Source: CAD feature listing. Evaluate the final solid. Frame: model axes, mm. A direction names the side the tool comes from. Give positions to 0.01 mm unless a question says otherwise; leave off trailing zeros. Order: outer loops, then holes, each group sorted by start corner. A loop starts at its lowest first (then second) coordinate and runs counter-clockwise, first axis right, second up.
from build123d import *

# Parameters (mm, degrees)
F0_R     = 40
F1_DEPTH = 120
F2_R     = 2.65
F3_DEPTH = 10
F4_R     = 2.25
F5_DEPTH = 25
F6_R     = 37.5
F7_DEPTH = 119
F8_R     = 39.694818
F9_DEPTH = 1


with BuildPart() as f1:
    # F0 (on Top) → F1 (new body)
    with BuildSketch(Plane.XY):
        with Locations((-32.717515, 13.759183)):
            Circle(F0_R)
    extrude(amount=F1_DEPTH)

    # F2 (on face) → F3 (join)
    with BuildSketch(Plane.XY.offset(120)):
        with Locations((-32.717515, 13.759183)):
            Circle(F2_R)
    extrude(amount=F3_DEPTH)

    # F4 (on face) → F5 (cut)
    with BuildSketch(Plane.XY.offset(130)):
        with Locations((-32.717515, 13.759183)):
            Circle(F4_R)
    extrude(amount=-F5_DEPTH, mode=Mode.SUBTRACT)

    # F6 (on face) → F7 (cut)
    with BuildSketch(Plane(origin=(0, 0, 0), x_dir=(1, 0, 0), z_dir=(0, 0, -1))):
        with Locations((-32.717515, -13.759183)):
            Circle(F6_R)
    extrude(amount=-F7_DEPTH, mode=Mode.SUBTRACT)

    # F8 (on Top) → F9 (join)
    with BuildSketch(Plane.XY):
        with Locations((-32.779191, 13.591371)):
            Circle(F8_R)
    extrude(amount=F9_DEPTH)


solid = f1.part
1) First-contact query: pin 1 Ø6 at (y, z) = (-5, 38.5) entering from +X; pin 2 Ø5 at (x, y) = (-33.5, 42) entering from +Z; pin 3 Ø6 at (x, z) = (-15.5, 50) entering from -Y. Flat tips, straight axial feed; report the tip coordinate or a pass-through.
Checks:
pin 1: stops at x = 4.05
pin 2: stops at z = 120
pin 3: stops at y = -23.63
2) Reachability of faces 4 (the face through (-70.18, 12.11, 59.17)), 5 (the face through (-34.376, 15.28, 124.577)), 6 (the face through (5.435, 25.774, 59.16)) from +Z, -Z, +X, -X, +Y, -Y: full face, straight path, thin tool, end or side. Return the list, or none.
Checks:
face 4: none
face 5: +Z
face 6: +Z, -Z
3) Section query B-B on y = -5. Output: boundary loops of the cut face in (x, z), and give its area (3 significant figures).
Checks:
outline: (-68.05, 0) - (2.61, 0) - (2.61, 120) - (-68.05, 120) - close; hole (-65.19, 1) - (-0.25, 1) - (-0.25, 119) - (-65.19, 119) - close
area: 816 mm2
4) Ray query, L1, parallel to Z at x = -20, y = 39.5; L2, parallel to Z at x = -31.5, y = 13; L3, parallel to Y at x = -54, z = 31. Return the intervals inside material, ascending.
Checks:
L1: z = 0 to 1, 119 to 120
L2: z = 0 to 1
L3: y = -20.11 to -17.12, 44.63 to 47.63
5) Section query C-C on z = 9. Output: boundary loops of the cut face in (x, y), and give its area (3 significant figures).
Checks:
outline: circle Ø80 at (-32.72, 13.76); hole circle Ø75 at (-32.72, 13.76)
area: 609 mm2
6) Pull-direction query (X, two-part tool) for faces 1 (the face through (-33, 22, 119)), 2 (the face through (-30.19, 14.56, 124.93)), 3 (the face through (-35, 13, 130)); classes: +X half, -X half, draft (parallel to the pull), parting line (faces both ways), or undercut.
Checks:
face 1: undercut
face 2: parting line
face 3: draft
7) Section query A-A on x = -7.5. Output: boundary loops of the cut face in (y, z).
Checks:
outline: (-17.29, 0) - (44.81, 0) - (44.81, 120) - (-17.29, 120) - close; hole (-14, 1) - (41.51, 1) - (41.51, 119) - (-14, 119) - close
